Autodesk Inventor part; units mm, degrees
ref_plane "YZ Plane" through (0, 0, 0) normal (1, 0, 0) x (0, 1, 0)
ref_plane "XZ Plane" through (0, 0, 0) normal (0, 1, 0) x (-1, 0, 0)
ref_plane "XY Plane" through (0, 0, 0) normal (0, 0, 1) x (1, 0, 0)
sketch "草图1" plane through (0, 0, 0) normal (0, 0, 1) x (1, 0, 0)
  circle A0 centre (-9.405, -0.7961) radius 2
  line L0 (-4.9391, -16.3471) -> (-4.9391, -13.3471)
  line L1 (-4.9391, -13.3471) -> (-6.4391, -13.3471)
  line L2 (-6.4391, -13.3471) -> (-6.4391, 13.6529)
  line L3 (-4.9391, 13.6529) -> (-6.4391, 13.6529)
  line L4 (-4.9391, 16.6529) -> (-4.9391, 13.6529)
  line L5 (-4.9391, 16.6529) -> (-11.9051, 16.6529)
  line L6 (-11.9051, 16.6529) -> (-11.9051, -16.3471)
  line L7 (-4.9391, -16.3471) -> (-11.9051, -16.3471)
  circle A1 centre (9.5269, -0.7961) radius 2
  line L8 (5.0609, -16.3471) -> (12.0269, -16.3471)
  line L9 (12.0269, -16.3471) -> (12.0269, 16.6529)
  line L10 (5.0609, 16.6529) -> (12.0269, 16.6529)
  line L11 (5.0609, 16.6529) -> (5.0609, 13.6529)
  line L12 (6.5609, 13.6529) -> (5.0609, 13.6529)
  line L13 (6.5609, -13.3471) -> (6.5609, 13.6529)
  line L14 (6.5609, -13.3471) -> (5.0609, -13.3471)
  line L15 (5.0609, -13.3471) -> (5.0609, -16.3471)
  line L16 (12.0269, -16.3471) -> (-11.9051, -16.3471)
  line L17 (-11.9051, -16.3471) -> (-11.9051, 16.6529)
  line L18 (-11.9051, 16.6529) -> (12.0269, 16.6529)
  line L19 (12.0269, 16.6529) -> (12.0269, -16.3471)
  circle A2 centre (9.5269, -0.7961) radius 1.5
  circle A3 centre (-9.405, -0.7961) radius 1.5
  dimension "d2" = 0.5
  dimension "d3" = 0.5
extrude "拉伸1" add sketch "草图1" along normal blind 2 contours A0 | L7 L6 L5 L4 L3 L2 L1 L0 | L0 L1 L2 L3 L4 L18 L11 L12 L13 L14 L15 L16 | L15 L14 L13 L12 L11 L10 L9 L8 | A1
properties part number "触点外壳"
Geometry: final body of the model. Coordinates: model frame, mm. Round coordinates to 2 decimals unless told otherwise and drop trailing zeros. Write each loop counter-clockwise with the first axis right and the second up, starting at its lowest first coordinate (ties: lowest second). Pieces come first, ordered by that corner, then holes.
Item 1: Section query A-A (x = -8.5). Return loops of the section in (y, z).
Item 2: Material intervals for L1, parallel to X at y = 0, z = 0.55; L2, parallel to Y at x = -9.5, z = 1.45; L3, parallel to Y at x = 10.5, z = 0.3, sorted ascending.
Item 3: Section query B-B (z = 1.35). Return loops of the section in (x, y) (3 decimals).
Item 4: Mould query, pull axis Y, two halves, no side actions, for faces 1 (the face through (0, 0, 2)), 2 (the face through (10.91, -0.22, 0.99)), 3 (the face through (0, -16.347, 1)). Classes: +Y half, -Y half, draft (parallel to the pull), parting line (faces both ways), or undercut.
Completed:
1. outline: (-16.35, 0) - (-1.99, 0) - (-1.99, 2) - (-16.35, 2) - close; (0.4, 0) - (16.65, 0) - (16.65, 2) - (0.4, 2) - close
2. L1: x = -11.91 to -10.68, -8.13 to 8.26, 10.8 to 12.03
2. L2: y = -16.35 to -2.29, 0.7 to 16.65
2. L3: y = -16.35 to -1.94, 0.35 to 16.65
3. outline: (-11.905, -16.347) - (12.027, -16.347) - (12.027, 16.653) - (-11.905, 16.653) - close; hole circle Ø3 at (-9.405, -0.796); hole circle Ø3 at (9.527, -0.796)
4. face 1: draft
4. face 2: undercut
4. face 3: -Y half
